Job drawing, mm, ordinate dimensions from the low corner. One solid piece. A direction names the side the tool comes from. Coordinates: 2 decimals unless noted, no trailing zeros. Loops run counter-clockwise (first coordinate to the right, second up) from the corner with the lowest first, then second, coordinate; pieces in that order, holes last. Notation, with made-up numbers: M -13.5,-28 L 27.5,-28 A20 ccw 27.5,-7 Z; hole C 80,-8.75 d3. An arc over 180 degrees is marked long. Write each question's results on one line, items separated by ' | '. Start each with the question number.
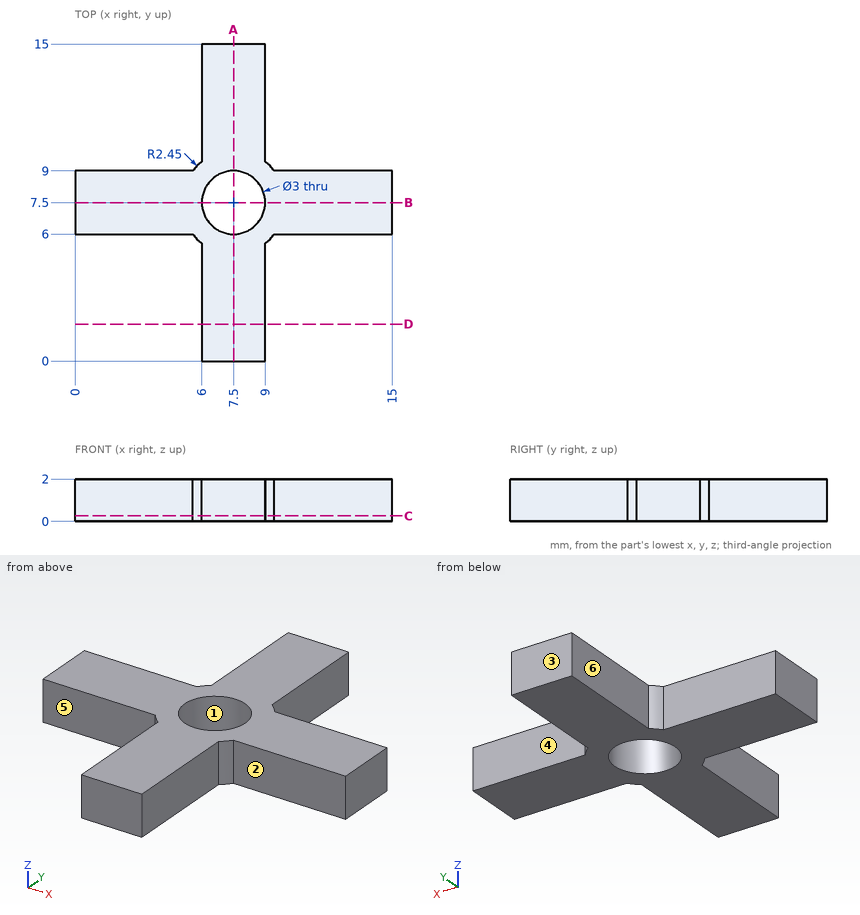
1. Wall check: line 1 along Y through (x, z) = (7.5, 1.3); line 2 along Y through (x, z) = (5.5, 0.55). Give the ranges that are in metal, low to high.
2. Which spindle directions (+Z, -Z, +X, -X, +Y, -Y) get a long thin tool onto all of the face, cutting with end or side? Do the marked faces 4, 5 and 6. Say none if no direction does.
3. Band-saw the part on A-A, the plane x = 7.5. List the corners of the cut face in (y, z), plus the area to 3 significant figures.
4. Band-saw the part on C-C, the plane z = 0.25. List the corners of the cut face in (x, y).
5. Band-saw the part on D-D, the plane y = 1.75. List the corners of the cut face in (x, z), plus the area to 3 significant figures.
6. Mould opens along Y. For the marked faces 1, 2 and 3 say: +Y half, -Y half, draft (parallel to the pull), parting line (faces both ways), or undercut.
7. Pin check, flat tips, straight feed: pin 1 (1 mm diameter, centred on x = 12.5, z = 1.5, fed in from -Y); pin 2 (1 mm diameter, centred on y = 13, z = 0.5, fed in from +X). Stop position of each tip, or through.
Checked values:
1) line 1: 0 to 6, 9 to 15 | line 2: 6 to 9
2) face 4: +Z, -Z, +X, +Y | face 5: +Z, -Z, -X, -Y | face 6: +Z, -Z, -X, +Y
3) outline: M 0,0 L 6,0 L 6,2 L 0,2 Z; M 9,0 L 15,0 L 15,2 L 9,2 Z | area: 24.0 mm²
4) outline: M 0,6 L 5.56,6 A2.45 ccw 6,5.56 L 6,0 L 9,0 L 9,5.56 A2.45 ccw 9.44,6 L 15,6 L 15,9 L 9.44,9 A2.45 ccw 9,9.44 L 9,15 L 6,15 L 6,9.44 A2.45 ccw 5.56,9 L 0,9 Z; hole C 7.5,7.5 d3
5) outline: M 6,0 L 9,0 L 9,2 L 6,2 Z | area: 6.00 mm²
6) face 1: undercut | face 2: -Y half | face 3: +Y half
7) pin 1: y = 6 | pin 2: x = 9
